Part model, mm, in its own coordinate system. A direction names the side the tool comes from. Coordinates: 2 decimals unless noted, no trailing zeros. Write each loop counter-clockwise with the first axis right and the second up, starting at its lowest first coordinate (ties: lowest second). Pieces come first, ordered by that corner, then holes. Notation, with made-up numbers: (52, -0.5) - (93, -0.5) arc R33 ccw to (93, 27.5) - close; hole circle Ø10 at (-37.75, 54.25). An arc over 180 degrees is marked (long way). Use a Markdown table: item, result.
```python
from build123d import *

# Parameters (mm, degrees)
BOX148_W          = 3
BOX148_H          = 6
BOX148_DEPTH      = 9
BOX149_W          = 3
BOX149_H          = 6
BOX149_DEPTH      = 9
BOX151_W          = 2
BOX151_H          = 10.25
BOX151_DEPTH      = 3
BOX152_W          = 2
BOX152_H          = 10.25
BOX152_DEPTH      = 3
BOX153_W          = 1
BOX153_H          = 10.25
BOX153_DEPTH      = 2
BOX154_W          = 1
BOX154_H          = 10.25
BOX154_DEPTH      = 2
BOX155_W          = 7.5
BOX155_H          = 5.5
BOX155_DEPTH      = 3
BOX156_W          = 9
BOX156_H          = 2
BOX156_DEPTH      = 3
BOX157_W          = 9
BOX157_H          = 2
BOX157_DEPTH      = 3
BOX158_W          = 10
BOX158_H          = 1
BOX158_DEPTH      = 2
BOX159_W          = 10
BOX159_H          = 1
BOX159_DEPTH      = 2
CYLINDER066_R     = 1.6
CYLINDER066_DEPTH = 3
BOX150_W          = 13.5
BOX150_H          = 6
BOX150_DEPTH      = 2.3
FILLET035_R       = 2
CYLINDER065_R     = 1.6
CYLINDER065_DEPTH = 1.5
CYLINDER064_R     = 1.6
CYLINDER064_DEPTH = 1.5
CYLINDER063_R     = 25.5
CYLINDER063_DEPTH = 3
CYLINDER062_R     = 25.5
CYLINDER062_DEPTH = 3
BOX147_W          = 45
BOX147_H          = 23
BOX147_DEPTH      = 1.5
FILLET034_R       = 5


with BuildPart() as cube137:
    # Box148 → Box148 (new body)
    with BuildSketch(Plane(origin=(52.5, 29.25, -3), x_dir=(1, 0, 0), z_dir=(0, 0, 1))):
        with Locations((1.5, 3)):
            Rectangle(BOX148_W, BOX148_H)
    extrude(amount=BOX148_DEPTH)


with BuildPart() as cube138:
    # Box149 → Box149 (new body)
    with BuildSketch(Plane(origin=(63, 29.25, -3), x_dir=(1, 0, 0), z_dir=(0, 0, 1))):
        with Locations((1.5, 3)):
            Rectangle(BOX149_W, BOX149_H)
    extrude(amount=BOX149_DEPTH)


with BuildPart() as cube140:
    # Box151 → Box151 (new body)
    with BuildSketch(Plane(origin=(41.5, 20, -3), x_dir=(1, 0, 0), z_dir=(0, 0, 1))):
        with Locations((1, 5.125)):
            Rectangle(BOX151_W, BOX151_H)
    extrude(amount=BOX151_DEPTH)


with BuildPart() as cube141:
    # Box152 → Box152 (new body)
    with BuildSketch(Plane(origin=(75, 20, -3), x_dir=(1, 0, 0), z_dir=(0, 0, 1))):
        with Locations((1, 5.125)):
            Rectangle(BOX152_W, BOX152_H)
    extrude(amount=BOX152_DEPTH)


with BuildPart() as cube142:
    # Box153 → Box153 (new body)
    with BuildSketch(Plane(origin=(41.5, 20, 0), x_dir=(1, 0, 0), z_dir=(0, 0, 1))):
        with Locations((0.5, 5.125)):
            Rectangle(BOX153_W, BOX153_H)
    extrude(amount=BOX153_DEPTH)


with BuildPart() as cube143:
    # Box154 → Box154 (new body)
    with BuildSketch(Plane(origin=(76, 20, 0), x_dir=(1, 0, 0), z_dir=(0, 0, 1))):
        with Locations((0.5, 5.125)):
            Rectangle(BOX154_W, BOX154_H)
    extrude(amount=BOX154_DEPTH)


with BuildPart() as cube144:
    # Box155 → Box155 (new body)
    with BuildSketch(Plane(origin=(55.5, 28.5, -3), x_dir=(1, 0, 0), z_dir=(0, 0, 1))):
        with Locations((3.75, 2.75)):
            Rectangle(BOX155_W, BOX155_H)
    extrude(amount=BOX155_DEPTH)


with BuildPart() as cube145:
    # Box156 → Box156 (new body)
    with BuildSketch(Plane(origin=(43.5, 28.25, -3), x_dir=(1, 0, 0), z_dir=(0, 0, 1))):
        with Locations((4.5, 1)):
            Rectangle(BOX156_W, BOX156_H)
    extrude(amount=BOX156_DEPTH)


with BuildPart() as cube146:
    # Box157 → Box157 (new body)
    with BuildSketch(Plane(origin=(66, 28.25, -3), x_dir=(1, 0, 0), z_dir=(0, 0, 1))):
        with Locations((4.5, 1)):
            Rectangle(BOX157_W, BOX157_H)
    extrude(amount=BOX157_DEPTH)


with BuildPart() as cube147:
    # Box158 → Box158 (new body)
    with BuildSketch(Plane(origin=(66, 29.25, 0), x_dir=(1, 0, 0), z_dir=(0, 0, 1))):
        with Locations((5, 0.5)):
            Rectangle(BOX158_W, BOX158_H)
    extrude(amount=BOX158_DEPTH)


with BuildPart() as cube148:
    # Box159 → Box159 (new body)
    with BuildSketch(Plane(origin=(42.5, 29.25, 0), x_dir=(1, 0, 0), z_dir=(0, 0, 1))):
        with Locations((5, 0.5)):
            Rectangle(BOX159_W, BOX159_H)
    extrude(amount=BOX159_DEPTH)


with BuildPart() as cylinder147:
    # Cylinder066 → Cylinder066 (new body)
    with BuildSketch(Plane(origin=(59.25, 32.25, 6), x_dir=(1, 0, 0), z_dir=(0, 0, 1))):
        Circle(CYLINDER066_R)
    extrude(amount=CYLINDER066_DEPTH)


with BuildPart() as cut090:
    # Box150 → Box150 (new body)
    with BuildSketch(Plane(origin=(52.5, 29.25, 6), x_dir=(1, 0, 0), z_dir=(0, 0, 1))):
        with Locations((6.75, 3)):
            Rectangle(BOX150_W, BOX150_H)
    extrude(amount=BOX150_DEPTH)

    # Fillet035
    fillet035_edges = [cut090.edges().sort_by_distance(p)[0] for p in [
        (52.5, 32.25, 8.3),
        (66, 32.25, 8.3),
    ]]
    fillet(fillet035_edges, radius=FILLET035_R)

    # Cut090: cut Cylinder147
    add(cylinder147.part, mode=Mode.SUBTRACT)


with BuildPart() as cylinder146:
    # Cylinder065 → Cylinder065 (new body)
    with BuildSketch(Plane(origin=(76.5, 33, -4.5), x_dir=(1, 0, 0), z_dir=(0, 0, 1))):
        Circle(CYLINDER065_R)
    extrude(amount=CYLINDER065_DEPTH)


with BuildPart() as cylinder145:
    # Cylinder064 → Cylinder064 (new body)
    with BuildSketch(Plane(origin=(42.5, 33, -4.5), x_dir=(1, 0, 0), z_dir=(0, 0, 1))):
        Circle(CYLINDER064_R)
    extrude(amount=CYLINDER064_DEPTH)


with BuildPart() as cylinder144:
    # Cylinder063 → Cylinder063 (new body)
    with BuildSketch(Plane(origin=(102, 14, -6), x_dir=(1, 0, 0), z_dir=(0, 0, 1))):
        Circle(CYLINDER063_R)
    extrude(amount=CYLINDER063_DEPTH)


with BuildPart() as cylinder143:
    # Cylinder062 → Cylinder062 (new body)
    with BuildSketch(Plane(origin=(16.5, 14, -6), x_dir=(1, 0, 0), z_dir=(0, 0, 1))):
        Circle(CYLINDER062_R)
    extrude(amount=CYLINDER062_DEPTH)


with BuildPart() as fusion049:
    # Box147 → Box147 (new body)
    with BuildSketch(Plane(origin=(37, 15, -4.5), x_dir=(1, 0, 0), z_dir=(0, 0, 1))):
        with Locations((22.5, 11.5)):
            Rectangle(BOX147_W, BOX147_H)
    extrude(amount=BOX147_DEPTH)

    # Cut086: cut Cylinder143
    add(cylinder143.part, mode=Mode.SUBTRACT)

    # Cut087: cut Cylinder144
    add(cylinder144.part, mode=Mode.SUBTRACT)

    # Fillet034
    fillet034_edges = [fusion049.edges().sort_by_distance(p)[0] for p in [
        (82, 38, -3.75),
        (37, 38, -3.75),
    ]]
    fillet(fillet034_edges, radius=FILLET034_R)

    # Cut088: cut Cylinder145
    add(cylinder145.part, mode=Mode.SUBTRACT)

    # Cut089: cut Cylinder146
    add(cylinder146.part, mode=Mode.SUBTRACT)

    # Fusion049: union Cube137, Cube138, Cube140, Cube141, Cube142, Cube143, Cube144, Cube145, Cube146, Cube147, Cube148, Cut090
    add(cube137.part)
    add(cube138.part)
    add(cube140.part)
    add(cube141.part)
    add(cube142.part)
    add(cube143.part)
    add(cube144.part)
    add(cube145.part)
    add(cube146.part)
    add(cube147.part)
    add(cube148.part)
    add(cut090.part)


solid = fusion049.part
```
Item 1: Which spindle directions (+Z, -Z, +X, -X, +Y, -Y) get a long thin tool onto all of the face, cutting with end or side? Do faces 5 (the face through (59, 15, -4)), 6 (the face through (47, 30.25, -1)), 7 (the face through (58, 34, 6)), 8 (the face through (48, 28.25, -2)), 9 (the face through (59.2, 35.25, 6.3)). Say none if no direction does.
From the geometry:
| item | result |
|---|---|
| face 5 | +Z, -Z, +X, -X, -Y |
| face 6 | +Z, -X, +Y |
| face 7 | +Y, -Y |
| face 8 | +Z, -Y |
| face 9 | +Z, +X, -X, +Y |
Item 2: Band-saw the part on B-B, the plane x = 59.25. Give the cut face in (y, z), then the cut area to 3 significant figures.
From the geometry:
| item | result |
|---|---|
| outline | (15, -4.5) - (38, -4.5) - (38, -3) - (34, -3) - (34, 0) - (28.5, 0) - (28.5, -3) - (15, -3) - close; (29.25, 6) - (30.65, 6) - (30.65, 8.3) - (29.25, 8.3) - close; (33.85, 6) - (35.25, 6) - (35.25, 8.3) - (33.85, 8.3) - close |
| area | 57.4 mm^2 |
Item 3: Band-saw the part on A-A, the plane z = 4. Give the cut face in (x, y).
From the geometry:
| item | result |
|---|---|
| outline | (52.5, 29.25) - (55.5, 29.25) - (55.5, 35.25) - (52.5, 35.25) - close; (63, 29.25) - (66, 29.25) - (66, 35.25) - (63, 35.25) - close |
Item 4: Band-saw the part on D-D, the plane x = 47. Give the cut face in (y, z), then the cut area to 3 significant figures.
From the geometry:
| item | result |
|---|---|
| outline | (15, -4.5) - (38, -4.5) - (38, -3) - (30.25, -3) - (30.25, 2) - (29.25, 2) - (29.25, 0) - (28.25, 0) - (28.25, -3) - (15, -3) - close |
| area | 42.5 mm^2 |
Item 5: Drop flat-ended pins along their axis: P1, Ø3, axis at x = 76.5, y = 33, coming from the +Z side; P2, Ø3.5, axis at x = 60, z = -1, coming from the +Y side; P3, Ø3, axis at y = 31, z = 1.5, coming from the -X side; P4, Ø3, axis at x = 75.5, z = 2.5, coming from the +Y side. Give the stop position or say it passes through.
From the geometry:
| item | result |
|---|---|
| P1 | through |
| P2 | y = 34 |
| P3 | x = 41.5 |
| P4 | y = 30.25 |
Item 6: Drill centre lines: probe 1 along Y at (x, z) = (59.25, 6.75); probe 2 along X at (y, z) = (25, 0.75); probe 3 along X at (y, z) = (31.75, -3.75). Where is each one in solid material? Low to high.
From the geometry:
| item | result |
|---|---|
| probe 1 | 29.25 to 30.65, 33.85 to 35.25 |
| probe 2 | 41.5 to 42.5, 76 to 77 |
| probe 3 | 37 to 41.5, 43.5 to 75.5, 77.5 to 82 |
Item 7: Band-saw the part on C-C, the plane y = 32.25. Give the cut face in (x, z).
From the geometry:
| item | result |
|---|---|
| outline | (37, -4.5) - (41.09, -4.5) - (41.09, -3) - (37, -3) - close; (43.91, -4.5) - (75.09, -4.5) - (75.09, -3) - (66, -3) - (66, 6.3) arc R2 ccw to (64, 8.3) - (60.85, 8.3) - (60.85, 6) - (63, 6) - (63, 0) - (55.5, 0) - (55.5, 6) - (57.65, 6) - (57.65, 8.3) - (54.5, 8.3) arc R2 ccw to (52.5, 6.3) - (52.5, -3) - (43.91, -3) - close; (77.91, -4.5) - (82, -4.5) - (82, -3) - (77.91, -3) - close |
Item 8: Two-plate mould, pull along X, no slides. Class faces 1 (the face through (59, 31, 0)), 2 (the face through (60.73, 31.64, 7.13)), 3 (the face through (59, 38, -4)), 4 (the face through (78.122, 22.95, -3.76)): pulls with the +X half, pulls with the -X half, needs draft (parallel to the pull), parting line crosses it, or undercut.
From the geometry:
| item | result |
|---|---|
| face 1 | undercut |
| face 2 | undercut |
| face 3 | needs draft |
| face 4 | pulls with the +X half |
